Solid Edge part; units mm, degrees
sketch "Sketch1" plane through (0, 0, 0) normal (0, -1, 0) x (1, 0, 0)
  line L0 (-45, -40) -> (45, -40)
  line L1 (45, -40) -> (45, 40)
  line L2 (45, 40) -> (-45, 40)
  line L3 (-45, 40) -> (-45, -40)
  dimension "D1" = 45
  dimension "D2" = 45
extrude "Protrusion1" add sketch "Sketch1" against normal blind 8
sketch "Sketch2" plane through (0, 0, 0) normal (0, -1, 0) x (1, 0, 0)
  circle A0 centre (-40, 30) radius 1.4
  circle A1 centre (-40, -30) radius 1.4
  circle A2 centre (40, -30) radius 1.4
  circle A3 centre (40, 30) radius 1.4
  dimension "D1" = 40
  dimension "D2" = 40
extrude "Cutout1" cut sketch "Sketch2" against normal through all
sketch "Sketch3" plane through (0, 0, 0) normal (0, -1, 0) x (1, 0, 0)
  circle A0 centre (-21, 16) radius 4
  circle A1 centre (-21, -16) radius 4
  circle A2 centre (21, -16) radius 4
  circle A3 centre (21, 16) radius 4
extrude "Extrusionsausschnitt_2" cut sketch "Sketch3" against normal blind 5
sketch "Sketch4" plane through (0, 0, 0) normal (0, -1, 0) x (1, 0, 0)
  circle A0 centre (-21, 16) radius 1.75
  circle A1 centre (-21, -16) radius 1.75
  circle A2 centre (21, -16) radius 1.75
  circle A3 centre (21, 16) radius 1.75
extrude "Cutout2" cut sketch "Sketch4" against normal through all
fillet "Verrundung_1" radius 4 4 edges at (-45, 4, 40) (45, 4, 40) (45, 4, -40) (-45, 4, -40)
chamfer "Fase_1" distance 0.5 angle 60 4 edges at (38.6, 0, 30) (-41.4, 0, 30) (-41.4, 0, -30) (38.6, 0, -30) measured on face at (-29.1, 0, 27.4667)
chamfer "Fase_2" distance 0.5 angle 60 4 edges at (-40, 8, 31.4) (40, 8, 31.4) (40, 8, -28.6) (-40, 8, -28.6) measured on face at (-29.1, 8, 27.4667)
chamfer "Fase_4" distance 0.5 angle 60 4 edges at (-21, 5, 14.25) (-21, 5, -17.75) (21, 5, 14.25) (21, 5, -17.75) measured on face at (-23.5867, 5, 18.7467) measured on face at (-23.5867, 5, -13.2533) measured on face at (18.4133, 5, 18.7467) measured on face at (18.4133, 5, -13.2533)
sketch "Sketch5" plane through (0, 8, 0) normal (0, 1, 0) x (1, 0, 0)
  line L0 (-45, 11) -> (-37, 11)
  line L1 (-37, 11) -> (-37, 18)
  line L2 (-37, 18) -> (-45, 18)
  line L3 (-45, 18) -> (-45, 11)
  dimension "D1" = 45
  dimension "D2" = 45
extrude "Extrusionsausprägung_2" add sketch "Sketch5" along normal blind 14
mirror "Mirror1" about plane through (0, 0, 0) normal (0, 0, 1) of "Extrusionsausprägung_2"
mirror "Mirror2" about plane through (0, 0, 0) normal (1, 0, 0) of "Extrusionsausprägung_2", "Mirror1"
properties material "Nylon, allgemein"
Read the model definition and answer for the solid it produces. Units are mm, in the model's axes. A direction names the side the tool comes from. Round coordinates to 2 decimals unless told otherwise and drop trailing zeros. Write each loop counter-clockwise with the first axis right and the second up, starting at its lowest first coordinate (ties: lowest second). Pieces come first, ordered by that corner, then holes. Notation, with made-up numbers: (85, -16) - (91, -16) arc R38 ccw to (91, 22) - close; hole circle Ø6 at (76.5, 69.25). An arc over 180 degrees is marked (long way). One line per question, with ' | ' between items. Start each with the question number.
1. For a pull along Z with two mould halves and no side action, classify faces 4 (the face through (1, 4, 40)), 5 (the face through (-22.29, 6.92, -14.82)), 6 (the face through (-37, 15, -14)), 7 (the face through (-23, 5, -18)) as +Z half, -Z half, draft (parallel to the pull), parting line (faces both ways), or undercut.
2. Section B-B (y = 3) is taken. Give the number of separate pieces and of enclosed holes in the cut face, and give its area (3 significant figures).
3. Section C-C (x = 21) is taken. Determine the outline of the cut face in (y, z).
4. Section D-D (y = 16.5) is taken. Determine the outline of the cut face in (x, z).
5. Find the intervals of material crossed by probe 1 along Z at (x, y) = (21, 6.7); probe 2 along Z at (x, y) = (-21, 2.2); probe 3 along X at (y, z) = (19, -15.5), in increasing order. Write a range as [from, to].
6. For faces 1 (the face through (-37, 15, 15)), 2 (the face through (-23, 5, 14)), 3 (the face through (45, 6, -1)), determine the directions among +Z, -Z, +X, -X, +Y, -Y from which every point of the face is accessible in a straight line to the end or side of a thin tool.
7. Each of these flat-tipped pins is pushed along its axis until it touches: pin 1 (9 mm diameter, centred on x = 39.5, y = 18, fed in from +Z); pin 2 (9 mm diameter, centred on x = -21, z = 16, fed in from +Y); pin 3 (9 mm diameter, centred on x = 23, z = -15.5, fed in from -Y); pin 4 (4 mm diameter, centred on x = -40, y = 17.5, fed in from -Z). Where does it stop, or does it pass through?
8. Section A-A (z = 16) is taken. Determine the outline of the cut face in (x, y).
Filled in:
1) face 4: +Z half | face 5: undercut | face 6: draft | face 7: undercut
2) separate pieces: 1 | enclosed holes: 8 | area: 6,960 mm²
3) outline: (0, -40) - (8, -40) - (8, -17.75) - (5.87, -17.75) - (5, -18.25) - (5, -20) - (0, -20) - close; (0, -12) - (5, -12) - (5, -13.75) - (5.87, -14.25) - (8, -14.25) - (8, 14.25) - (5.87, 14.25) - (5, 13.75) - (5, 12) - (0, 12) - close; (0, 20) - (5, 20) - (5, 18.25) - (5.87, 17.75) - (8, 17.75) - (8, 40) - (0, 40) - close
4) outline: (-45, -18) - (-37, -18) - (-37, -11) - (-45, -11) - close; (-45, 11) - (-37, 11) - (-37, 18) - (-45, 18) - close; (37, -18) - (45, -18) - (45, -11) - (37, -11) - close; (37, 11) - (45, 11) - (45, 18) - (37, 18) - close
5) probe 1: [-40, -17.75], [-14.25, 14.25], [17.75, 40] | probe 2: [-40, -20], [-12, 12], [20, 40] | probe 3: [-45, -37], [37, 45]
6) face 1: +Z, -Z, +Y | face 2: -Y | face 3: +Z, -Z, +X, +Y, -Y
7) pin 1: z = 18 | pin 2: y = 8 | pin 3: y = 0 | pin 4: z = -18
8) outline: (-45, 0) - (-25, 0) - (-25, 5) - (-23.25, 5) - (-22.75, 5.87) - (-22.75, 8) - (-37, 8) - (-37, 22) - (-45, 22) - close; (-19.25, 5.87) - (-18.75, 5) - (-17, 5) - (-17, 0) - (17, 0) - (17, 5) - (18.75, 5) - (19.25, 5.87) - (19.25, 8) - (-19.25, 8) - close; (22.75, 5.87) - (23.25, 5) - (25, 5) - (25, 0) - (45, 0) - (45, 22) - (37, 22) - (37, 8) - (22.75, 8) - close
